from build123d import *

# Parameters (mm, degrees)
SKETCH1_W                      = 3
SKETCH1_H                      = 15
BOSS_EXTRUDE1_DEPTH            = 20.225
BOSS_EXTRUDE1_2_DEPTH          = 20.225
SKETCH2_W                      = 40
SKETCH2_H                      = 40
BOSS_EXTRUDE2_DEPTH            = 5
M3_CLEARANCE_HOLE1_D           = 3.4
FILLET1_R                      = 7.5
FILLET3_R                      = 1
CBORE_FOR_M3_SHCS1_D           = 3.4
CBORE_FOR_M3_SHCS1_CBORE_D     = 6.5
CBORE_FOR_M3_SHCS1_CBORE_DEPTH = 3
FILLET5_R                      = 3


with BuildPart() as part:
    # Sketch1 → Boss-Extrude1 (new body)
    with BuildSketch(Plane(origin=(0, 0, 0), x_dir=(1, 0, 0), z_dir=(0, 1, 0))):
        with Locations((-3.075, 0)):
            Rectangle(SKETCH1_W, SKETCH1_H)
    extrude(amount=BOSS_EXTRUDE1_DEPTH)



with BuildPart() as body_2:
    # Sketch1 → Boss-Extrude1 2 (new body)
    with BuildSketch(Plane(origin=(0, 0, 0), x_dir=(1, 0, 0), z_dir=(0, 1, 0))):
        with Locations((3.075, 0)):
            Rectangle(SKETCH1_W, SKETCH1_H)
    extrude(amount=BOSS_EXTRUDE1_2_DEPTH)


with BuildPart() as part_1:
    add(part.part)

    add(body_2.part)  # Boss-Extrude2 merges body 2
    # Sketch2 → Boss-Extrude2 (add)
    with BuildSketch(Plane(origin=(0, 20.225, 0), x_dir=(1, 0, 0), z_dir=(0, 1, 0))):
        Rectangle(SKETCH2_W, SKETCH2_H)
    extrude(amount=BOSS_EXTRUDE2_DEPTH)

    # M3 Clearance Hole1 (through all)
    with Locations(Plane.ZY.offset(4.575)):
        with Locations((0, 11), (0, 4)):
            Hole(M3_CLEARANCE_HOLE1_D / 2)

    # Fillet1
    fillet1_edges = [part_1.edges().sort_by_distance(p)[0] for p in [
        (3.075, 0, 7.5),
        (-3.075, 0, 7.5),
        (-3.075, 0, -7.5),
        (3.075, 0, -7.5),
    ]]
    fillet(fillet1_edges, radius=FILLET1_R - 0.0001)  # a hair under: the kernel refuses the full size

    # Fillet3
    fillet3_edges = [part_1.edges().sort_by_distance(p)[0] for p in [
        (-3.075, 20.225, -7.5),
        (4.575, 13.86245, 7.5),
        (4.575, 13.86245, -7.5),
        (3.075, 20.225, 7.5),
        (4.575, 20.225, 0),
        (3.075, 20.225, -7.5),
        (-4.575, 20.225, 0),
        (4.575, 2.196669852, -5.303330148),
        (4.575, 2.196669852, 5.303330148),
        (-4.575, 2.196669852, -5.303330148),
        (-4.575, 2.196669852, 5.303330148),
        (-4.575, 13.86245, -7.5),
        (-4.575, 13.86245, 7.5),
        (-3.075, 20.225, 7.5),
    ]]
    fillet(fillet3_edges, radius=FILLET3_R)

    # CBORE for M3 SHCS1 (through all)
    with Locations(Plane(origin=(0, 20.225, 0), x_dir=(-1, 0, 0), z_dir=(0, -1, 0))):
        with Locations((-13, -13), (-13, 13), (13, 13), (13, -13)):
            CounterBoreHole(CBORE_FOR_M3_SHCS1_D / 2, CBORE_FOR_M3_SHCS1_CBORE_D / 2, CBORE_FOR_M3_SHCS1_CBORE_DEPTH)

    # Fillet5
    fillet5_edges = [part_1.edges().sort_by_distance(p)[0] for p in [
        (-20, 20.225, 0),
        (-20, 22.725, -20),
        (0, 20.225, 20),
        (-20, 22.725, 20),
        (20, 20.225, 0),
        (20, 22.725, 20),
        (0, 20.225, -20),
        (20, 22.725, -20),
    ]]
    fillet(fillet5_edges, radius=FILLET5_R)


solid = part_1.part
Here's how the part is built. I have some questions about the finished solid (model axes, mm). A direction names the side the tool comes from. Coordinates: 2 decimals unless noted, no trailing zeros. Write each loop counter-clockwise with the first axis right and the second up, starting at its lowest first coordinate (ties: lowest second). Pieces come first, ordered by that corner, then holes.
1) If we section it at C-C (y = 11): List the corners of the cut face in (x, z) for me (3 decimals).
Filled in:
outline: (-4.575, -6.5) arc R1 ccw to (-3.575, -7.5) - (-1.575, -7.5) - (-1.575, -1.7) - (-4.575, -1.7) - close; (-4.575, 1.7) - (-1.575, 1.7) - (-1.575, 7.5) - (-3.575, 7.5) arc R1 ccw to (-4.575, 6.5) - close; (1.575, -7.5) - (3.575, -7.5) arc R1 ccw to (4.575, -6.5) - (4.575, -1.7) - (1.575, -1.7) - close; (1.575, 1.7) - (4.575, 1.7) - (4.575, 6.5) arc R1 ccw to (3.575, 7.5) - (1.575, 7.5) - close
2) Which directions (+Z, -Z, +X, -X, +Y, -Y) give clear straight access to the entire face, cutting with the end or side of a thin tool? Please do faces 1 (the face through (3, 13, -7.5)), 2 (the face through (15.395, 21.704, 10.803)), 3 (the face through (1.575, 10, -2)).
Filled in:
face 1: -Z, +X, -X, -Y
face 2: -Y
face 3: +Z, -Z, -Y
3) If we section it at B-B (x = 13): List the corners of the cut face in (y, z) for me (3 decimals), plus the area to 3 significant figures.
Filled in:
outline: (20.225, -17) arc R3 ccw to (23.225, -20) - (25.225, -20) - (25.225, -14.7) - (23.225, -14.7) - (23.225, -16.25) - (20.225, -16.25) - close; (20.225, -9.75) - (23.225, -9.75) - (23.225, -11.3) - (25.225, -11.3) - (25.225, 11.3) - (23.225, 11.3) - (23.225, 9.75) - (20.225, 9.75) - close; (20.225, 16.25) - (23.225, 16.25) - (23.225, 14.7) - (25.225, 14.7) - (25.225, 20) - (23.225, 20) arc R3 ccw to (20.225, 17) - close
area: 144 mm2
4) If we section it at A-A (z = 13): List the corners of the cut face in (x, y) for me (3 decimals).
Filled in:
outline: (-20, 23.225) arc R3 ccw to (-17, 20.225) - (-16.25, 20.225) - (-16.25, 23.225) - (-14.7, 23.225) - (-14.7, 25.225) - (-20, 25.225) - close; (-11.3, 23.225) - (-9.75, 23.225) - (-9.75, 20.225) - (9.75, 20.225) - (9.75, 23.225) - (11.3, 23.225) - (11.3, 25.225) - (-11.3, 25.225) - close; (14.7, 23.225) - (16.25, 23.225) - (16.25, 20.225) - (17, 20.225) arc R3 ccw to (20, 23.225) - (20, 25.225) - (14.7, 25.225) - close
5) Thinking about a two-plate mould opening in Z: for faces 4 (the face through (0, 25.225, 0)), 5 (the face through (-3.05, 2.34, 0.37)), 6 (the face through (-19.14, 24.24, -19.1)), which applies, +Z half, -Z half, draft (parallel to the pull), parting line (faces both ways), or undercut?
Filled in:
face 4: draft
face 5: undercut
face 6: -Z half
6) I'm going to push flat-ended pins straight in: pin 1 (3 mm diameter, centred on x = 13, z = -13, fed in from +Y); pin 2 (6 mm diameter, centred on y = 17, z = 0, fed in from +X); pin 3 (0.6 mm diameter, centred on x = 3, y = 12.5, fed in from +Z); pin 4 (7 mm diameter, centred on x = -13.5, z = 12.5, fed in from -Y) (3 decimals). Where does each tip first touch, or does it pass through?
Filled in:
pin 1: passes through
pin 2: stops at x = 4.94
pin 3: stops at z = 7.5
pin 4: stops at y = 20.225
7) If I drill on line 1 (Y direction, x = -2.4, z = 0) (3 decimals); line 2 (X direction, y = 24.5, z = 13), over which ranges is the centre line in solid material (lowest first)?
Filled in:
line 1: y = 0 to 2.3, 5.7 to 9.3, 12.7 to 25.225
line 2: x = -20 to -14.7, -11.3 to 11.3, 14.7 to 20
8) If we section it at D-D (x = 0): List the corners of the cut face in (y, z) for me (3 decimals), plus the area to 3 significant figures.
Filled in:
outline: (20.225, -17) arc R3 ccw to (23.225, -20) - (25.225, -20) - (25.225, 20) - (23.225, 20) arc R3 ccw to (20.225, 17) - close
area: 196 mm2
